from build123d import *

# Parameters (mm, degrees)
SKETCH1_W           = 8
SKETCH1_H           = 22
BOSS_EXTRUDE1_DEPTH = 15
SKETCH2_R           = 1.75
CUT_EXTRUDE1_DEPTH  = 16
SKETCH3_R           = 3.25
CUT_EXTRUDE2_DEPTH  = 3.5


with BuildPart() as part:
    # Sketch1 → Boss-Extrude1 (new body)
    with BuildSketch(Plane.XY):
        with Locations((-4, -3.701030928)):
            Rectangle(SKETCH1_W, SKETCH1_H)
    extrude(amount=BOSS_EXTRUDE1_DEPTH)

    # Sketch2 → Cut-Extrude1 (cut, through all)
    with BuildSketch(Plane.XY.offset(15)):
        with Locations((-4, 2.298969072)):
            Circle(SKETCH2_R)
        with Locations((-4, -9.701030928)):
            Circle(SKETCH2_R)
    extrude(amount=-CUT_EXTRUDE1_DEPTH, mode=Mode.SUBTRACT)

    # Sketch3 → Cut-Extrude2 (cut)
    with BuildSketch(Plane.XY.offset(15)):
        with Locations((-4, 2.298969072)):
            Circle(SKETCH3_R)
        with Locations((-4, -9.701030928)):
            Circle(SKETCH3_R)
    extrude(amount=-CUT_EXTRUDE2_DEPTH, mode=Mode.SUBTRACT)


solid = part.part
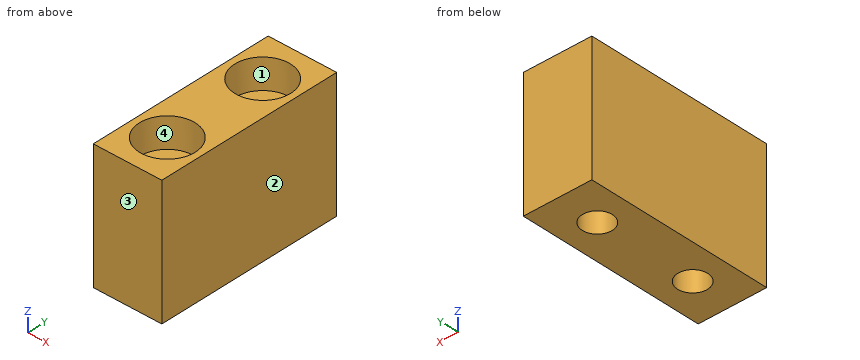
For this review, take the finished solid that the model builds, in its own axes (mm). Face numbers are marked on the shaded views. Round coordinates to 2 decimals unless told otherwise and drop trailing zeros. Order: outer loops, then holes, each group sorted by start corner. A loop starts at its lowest first (then second) coordinate and runs counter-clockwise, first axis right, second up. Notation, with made-up numbers: M 37.25,-30 L 93.25,-30 A37 ccw 93.25,8 Z; hole C 48,-8.5 d7. An arc over 180 degrees is marked long. Write each question's results on one line, items separated by ' | '. Start each with the question number.
1. Add section D-D (y = 5). State the section outline as (x, z) points, then the cut area to 3 significant figures.
2. To check wall thickness, follow L1, parallel to Y at x = -4, z = 9; L2, parallel to Y at x = -4, z = 12.55; L3, parallel to Z at x = -3.75, y = 0. State the ranges of each line that lie inside material, in increasing order. Write a range as [from, to].
3. Add section C-C (z = 12). State the section outline as (x, y) points, then the cut area to 3 significant figures.
4. Draft analysis for pull direction X (two halves, no side actions). For the marked faces 1, 2, 3 and 4, state which applies: pulls with the +X half, pulls with the -X half, needs draft (parallel to the pull), parting line crosses it, or undercut.
5. Clearance check with flat-ended pins moving along their axes: pin 1 Ø3 at (x, y) = (-4, -8.5) entering from +Z; pin 2 Ø3 at (x, y) = (-4, 2.3) entering from -Z. State where each tip first meets the part, or that it passes through.
6. Add section B-B (y = -8.25). State the section outline as (x, z) points.
7. Add section A-A (x = -4). State the section outline as (y, z) points, then the cut area to 3 significant figures.
Output values:
1) outline: M -8,0 L 0,0 L 0,15 L -2.19,15 L -2.19,11.5 L -5.81,11.5 L -5.81,15 L -8,15 Z | area: 107 mm^2
2) L1: [-14.7, -11.45], [-7.95, 0.55], [4.05, 7.3] | L2: [-14.7, -12.95], [-6.45, -0.95], [5.55, 7.3] | L3: [0, 11.5]
3) outline: M -8,-14.7 L 0,-14.7 L 0,7.3 L -8,7.3 Z; hole C -4,-9.7 d6.5; hole C -4,2.3 d6.5 | area: 110 mm^2
4) face 1: undercut | face 2: pulls with the +X half | face 3: needs draft | face 4: undercut
5) pin 1: z = 11.5 | pin 2: through
6) outline: M -8,0 L -4.98,0 L -4.98,11.5 L -6.91,11.5 L -6.91,15 L -8,15 Z; M -3.02,0 L 0,0 L 0,15 L -1.09,15 L -1.09,11.5 L -3.02,11.5 Z
7) outline: M -14.7,0 L -11.45,0 L -11.45,11.5 L -12.95,11.5 L -12.95,15 L -14.7,15 Z; M -7.95,0 L 0.55,0 L 0.55,11.5 L -0.95,11.5 L -0.95,15 L -6.45,15 L -6.45,11.5 L -7.95,11.5 Z; M 4.05,0 L 7.3,0 L 7.3,15 L 5.55,15 L 5.55,11.5 L 4.05,11.5 Z | area: 204 mm^2
